Source: CAD feature listing. Evaluate the final solid. Frame: model axes, mm. Face numbers are marked on the shaded views. A direction names the side the tool comes from. Round coordinates to 2 decimals unless told otherwise and drop trailing zeros. Order: outer loops, then holes, each group sorted by start corner. A loop starts at its lowest first (then second) coordinate and runs counter-clockwise, first axis right, second up. Notation, with made-up numbers: (-32.5, 51) - (10.5, 51) arc R13 ccw to (10.5, 64) - close; hole circle Ø6 at (31, 7). An arc over 180 degrees is marked (long way). Return JSON: item names as keys, results as strings. Group by question number.
1) Access query for the marked faces 1 and 2. Directions: +Z, -Z, +X, -X, +Y, -Y. A direction counts if a zero-diameter tool reaches every point of the face in a straight line with its end or side. Return the directions, or none.
2) Section A-A, the plane z = -4. Return loops of the section in (x, y), plus the area to 3 significant figures.
3) Section C-C, the plane x = 51.5. Return loops of the section in (y, z).
4) Section D-D, the plane z = -9.75. Return loops of the section in (x, y), plus the area to 3 significant figures.
5) Ray query, line 1 (Z direction, x = 29, y = -18.5); line 2 (Z direction, x = 64.5, y = -19). Return the intervals inside material, ascending. Write a range as from..to.
6) Contact query for flat-ended pins moving along their axis: P1, Ø4, axis at y = -10.5, z = -11, coming from the +X side; P2, Ø0.6, axis at y = 4, z = -12.5, coming from the +X side; P3, Ø1.5, axis at x = 47, y = 3.5, coming from the -Z side; P4, Ø1.5, axis at y = -11, z = -9.5, coming from the +X side. Output: stop coordinate, or through.
7) Section B-B, the plane y = -38. Return loops of the section in (x, z), plus the area to 3 significant figures.
```python
from build123d import *

# Parameters (mm, degrees)
PAD033_DEPTH    = 1
SKETCH055_W     = 8.1
SKETCH055_H     = 3.05
SKETCH055_W_2   = 3.05
SKETCH055_H_2   = 8.1
POCKET022_DEPTH = 0.5
POCKET023_DEPTH = 0.25
SKETCH057_W     = 3
SKETCH057_H     = 8
PAD034_DEPTH    = 0.5
SKETCH058_R     = 1.6
SKETCH058_R_2   = 1.97
PAD035_DEPTH    = 3.5
SKETCH059_W     = 9
SKETCH059_H     = 4
PAD036_DEPTH    = 12
SKETCH060_R     = 1.97
POCKET024_DEPTH = 31.34125859
CHAMFER009_SIZE = 1


with BuildPart() as part:
    # Sketch054 (on Face2 of Binder015) → Pad033 (new body)
    with BuildSketch(Plane(origin=(0, 0, -13), x_dir=(1, 0, 0), z_dir=(0, 0, -1))):
        Polygon((65.65, 44.999997), (65.65, 7.016667), (78, -5.333333), (13, -5.333333), (3.5165956595, 4.1500713405), (-2.14025859, 9.80692559), (-2.14025859, 44.999997), (13.05974141, 44.999997), (13.05974141, 47.899997), (27.95974141, 47.899997), (27.95974141, 44.999997), (40.05, 44.999997), (40.05, 47.899997), (54.95, 47.899997), (54.95, 44.999997), align=None)
    extrude(amount=-PAD033_DEPTH)

    # Sketch055 (on Face14 of Pad033) → Pocket022 (cut)
    with BuildSketch(Plane(origin=(0, 0, -13), x_dir=(1, 0, 0), z_dir=(0, 0, -1))):
        with Locations((22.5, -3.808333)):
            Rectangle(SKETCH055_W, SKETCH055_H)
        with Locations((45.5, -3.808333)):
            Rectangle(SKETCH055_W, SKETCH055_H)
        with Locations((68.5, -3.808333)):
            Rectangle(SKETCH055_W, SKETCH055_H)
        with Locations((64.125, 15.999997)):
            Rectangle(SKETCH055_W_2, SKETCH055_H_2)
        with Locations((64.125, 35.999997)):
            Rectangle(SKETCH055_W_2, SKETCH055_H_2)
        Polygon((71.6957629791, 0.9709040209), (69.5390872965, -1.1857716618), (63.8115223689, 4.5417932658), (65.9681980515, 6.6984689485), align=None)
        Polygon((11.119095962, -3.452428962), (5.3915310344, 2.2751359656), (7.5482067171, 4.4318116482), (13.2757716447, -1.2957532794), align=None)
    extrude(amount=-POCKET022_DEPTH, mode=Mode.SUBTRACT)

    # Sketch056 (on Face10 of Pocket022) → Pocket023 (cut)
    with BuildSketch(Plane.XY.offset(-12)):
        Polygon((65.65, -15.116667), (40.65, -15.116667), (14.9937160062, -29.9293294702), (-2.14025859, -29.9293294702), (-2.14025859, -29.4293294702), (14.85974141, -29.4293294702), (40.5160254038, -14.616667), (65.65, -14.616667), align=None)
    extrude(amount=-POCKET023_DEPTH, mode=Mode.SUBTRACT)

    # Sketch057 (on Face2 of Pocket023) → Pad034 (join)
    with BuildSketch(Plane(origin=(0, 0, -13), x_dir=(1, 0, 0), z_dir=(0, 0, -1))):
        with Locations((-3.64025859, 16.80692559)):
            Rectangle(SKETCH057_W, SKETCH057_H)
        with Locations((-3.64025859, 37.999997)):
            Rectangle(SKETCH057_W, SKETCH057_H)
        Polygon((1.0417219254, 6.6249450746), (-1.7867051994, 9.4533721994), (-3.9080255429, 7.3320518558), (-1.0795984182, 4.5036247311), align=None)
    extrude(amount=-PAD034_DEPTH)

    # Sketch058 (on Face9 of Pad034) → Pad035 (join)
    with BuildSketch(Plane.XY.offset(-12)):
        with Locations((25.85, -0.796667)):
            Circle(SKETCH058_R)
        with Locations((38.05, -0.796667)):
            Circle(SKETCH058_R_2)
    extrude(amount=PAD035_DEPTH)

    # Sketch059 (on Face10 of Pad035) → Pad036 (join)
    with BuildSketch(Plane.XY.offset(-12)):
        with Locations((6.99974141, -24.00692559)):
            Rectangle(SKETCH059_W, SKETCH059_H)
    extrude(amount=PAD036_DEPTH)

    # Sketch060 (on Face57 of Pad036) → Pocket024 (cut, through all)
    with BuildSketch(Plane.XZ.offset(26.00692559)):
        with Locations((6.99974141, -4)):
            Circle(SKETCH060_R)
    extrude(amount=-POCKET024_DEPTH, mode=Mode.SUBTRACT)

    # Chamfer009
    chamfer009_edges = [part.edges().sort_by_distance(p)[0] for p in [
        (2.499741, -26.006926, -6),
        (2.499741, -22.006926, -6),
        (2.499741, -24.006926, 0),
        (6.999741, -22.006926, 0),
        (11.499741, -24.006926, 0),
        (6.999741, -26.006926, 0),
        (11.499741, -26.006926, -6),
        (11.499741, -22.006926, -6),
    ]]
    chamfer(chamfer009_edges, length=CHAMFER009_SIZE)


solid = part.part
```
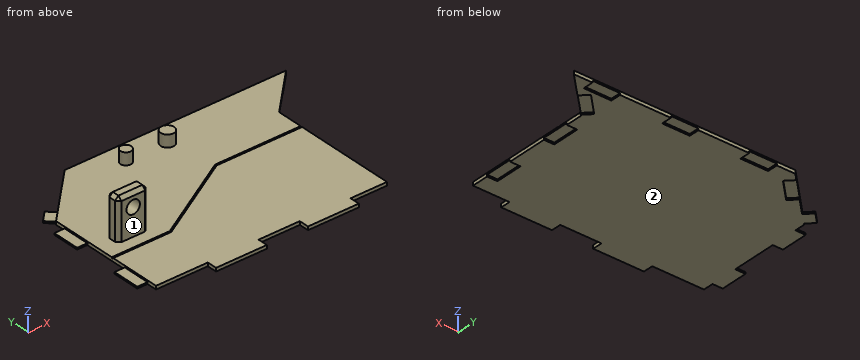
Geometry check:
{
 "1": {"face 1": "+Z, +X, -X, -Y", "face 2": "-Z, +X, -X, +Y, -Y"},
 "2": {"outline": "(2.5, -25.01) - (3.5, -26.01) - (5.03, -26.01) - (5.03, -22.01) - (3.5, -22.01) - (2.5, -23.01) - close; (8.97, -26.01) - (10.5, -26.01) - (11.5, -25.01) - (11.5, -23.01) - (10.5, -22.01) - (8.97, -22.01) - close", "area": "18.2 mm2"},
 "3": {"outline": "(-47.9, -13) - (5.33, -13) - (5.33, -12) - (-14.62, -12) - (-14.62, -12.25) - (-15.12, -12.25) - (-15.12, -12) - (-47.9, -12) - close"},
 "4": {"outline": "(2.5, -25.01) - (3.5, -26.01) - (10.5, -26.01) - (11.5, -25.01) - (11.5, -23.01) - (10.5, -22.01) - (3.5, -22.01) - (2.5, -23.01) - close; circle Ø3.2 at (25.85, -0.8); circle Ø3.94 at (38.05, -0.8)", "area": "54.2 mm2"},
 "5": {"line 1": "-13..-12", "line 2": "-12.5..-12"},
 "6": {"P1": "x = 65.65", "P2": "x = 76.97", "P3": "z = -12.5", "P4": "through"},
 "7": {"outline": "(-5.14, -13) - (62.6, -13) - (62.6, -12.5) - (65.65, -12.5) - (65.65, -12) - (-2.14, -12) - (-2.14, -12.5) - (-5.14, -12.5) - close", "area": "67.8 mm2"}
}
